Verification items for the finished model (mm, model axes). Face numbers are marked on the shaded views. A direction names the side the tool comes from. Coordinates: 2 decimals unless noted, no trailing zeros. Write each loop counter-clockwise with the first axis right and the second up, starting at its lowest first coordinate (ties: lowest second). Pieces come first, ordered by that corner, then holes. Notation, with made-up numbers: M 50,23 L 66,23 A13 cw 66,44 Z; hole C -27,6 d3. An arc over 180 degrees is marked long. Answer in a Markdown table with one row per item.
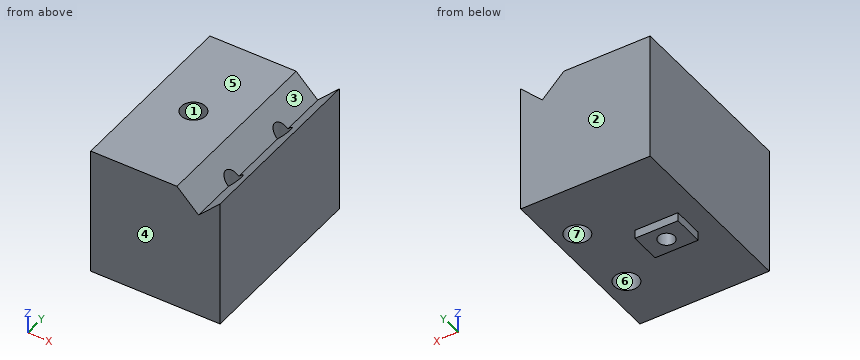
from build123d import *

# Parameters (mm, degrees)
F0_W      = 76.2
F0_H      = 76.2
F1_DEPTH  = 53.975
F3_DEPTH  = 107.951
F5_W      = 18.288
F5_H      = 5.08
F6_DEPTH  = 63.5
F4_R      = 4.7625
F7_DEPTH  = 81.281
F8_R      = 7.1501
F9_DEPTH  = 12.7
F10_R     = 7.1501
F11_DEPTH = 12.7
F12_W     = 38.1
F12_H     = 9
F13_DEPTH = 107.951


with BuildPart() as f1:
    # F0 (on Front) → F1 (new body, symmetric)
    with BuildSketch(Plane.XZ):
        with Locations((0, 38.1)):
            Rectangle(F0_W, F0_H)
    extrude(amount=F1_DEPTH, both=True)

    # F2 (on face) → F3 (cut, through all)
    with BuildSketch(Plane.XZ.offset(53.975)):
        Polygon((38.1, 76.2), (12.7, 76.2), (25.4, 63.5), align=None)
    extrude(amount=-F3_DEPTH, mode=Mode.SUBTRACT)

    # F5 (on face) → F6 (join)
    with BuildSketch(Plane.YZ.offset(38.1)):
        with Locations((0, -2.54)):
            Rectangle(F5_W, F5_H)
    extrude(amount=-F6_DEPTH)

    # F4 (on face) → F7 (cut, through all)
    with BuildSketch(Plane.XY.offset(76.2)):
        with Locations((25.4, 22.225)):
            Circle(F4_R)
        with Locations((25.4, -22.225)):
            Circle(F4_R)
        with Locations((-12.7, 0)):
            Circle(F4_R)
    extrude(amount=-F7_DEPTH, mode=Mode.SUBTRACT)

    # F8 (on face) → F9 (cut)
    with BuildSketch(Plane(origin=(0, 0, 0), x_dir=(1, 0, 0), z_dir=(0, 0, -1))):
        with Locations((25.4, -22.225)):
            Circle(F8_R)
        with Locations((25.4, 22.225)):
            Circle(F8_R)
    extrude(amount=-F9_DEPTH, mode=Mode.SUBTRACT)

    # F10 (on face) → F11 (cut)
    with BuildSketch(Plane.XY.offset(76.2)):
        with Locations((-12.7, 0)):
            Circle(F10_R)
    extrude(amount=-F11_DEPTH, mode=Mode.SUBTRACT)

    # F12 (on face) → F13 (cut, through all)
    with BuildSketch(Plane.XZ.offset(53.975)):
        with Locations((19.05, -4.5)):
            Rectangle(F12_W, F12_H)
    extrude(amount=-F13_DEPTH, mode=Mode.SUBTRACT)


solid = f1.part
1) Release check for a two-part mould opening along Y. For the marked faces 4, 5, 6 and 7 record: +Y half, -Y half, draft (parallel to the pull), parting line (faces both ways), or undercut.
Response values:
| item | result |
|---|---|
| face 4 | -Y half |
| face 5 | draft |
| face 6 | undercut |
| face 7 | undercut |
2) Sectioned sample at D-D (x = -21.5). Record the cut outline in (y, z) (3 decimals).
Response values:
| item | result |
|---|---|
| outline | M -53.975,0 L -9.144,0 L -9.144,-5.08 L 9.144,-5.08 L 9.144,0 L 53.975,0 L 53.975,76.2 L -53.975,76.2 Z |
3) Depth check by flat-ended pin: pin 1 (2.5 mm diameter, centred on y = -2, z = -2.5, fed in from -X); pin 2 (4.5 mm diameter, centred on x = 27.5, y = -19.5, fed in from -Z); pin 3 (15 mm diameter, centred on x = -12.7, y = 0, fed in from +Z); pin 4 (1.5 mm diameter, centred on x = 19.5, y = 16.5, fed in from -Z). Enter the tip coordinate at first touch or a pass-through.
Response values:
| item | result |
|---|---|
| pin 1 | stops at x = -25.4 |
| pin 2 | stops at z = 12.7 |
| pin 3 | stops at z = 76.2 |
| pin 4 | stops at z = 0 |
4) Sectioned sample at C-C (x = -12.7). Record the cut outline in (y, z) (1 decimal).
Response values:
| item | result |
|---|---|
| outline | M -54,0 L -9.1,0 L -9.1,-5.1 L -4.8,-5.1 L -4.8,63.5 L -7.2,63.5 L -7.2,76.2 L -54,76.2 Z; M 4.8,-5.1 L 9.1,-5.1 L 9.1,0 L 54,0 L 54,76.2 L 7.2,76.2 L 7.2,63.5 L 4.8,63.5 Z |
5) Sectioned sample at A-A (y = 0). Record the cut outline in (x, z).
Response values:
| item | result |
|---|---|
| outline | M -38.1,0 L -25.4,0 L -25.4,-5.08 L -17.46,-5.08 L -17.46,63.5 L -19.85,63.5 L -19.85,76.2 L -38.1,76.2 Z; M -7.94,-5.08 L 0,-5.08 L 0,0 L 38.1,0 L 38.1,76.2 L 25.4,63.5 L 12.7,76.2 L -5.55,76.2 L -5.55,63.5 L -7.94,63.5 Z |
6) Sectioned sample at B-B (z = 65). Record the cut outline in (x, y) (1 decimal), then the cut area to 4 significant figures.
Response values:
| item | result |
|---|---|
| outline | M -38.1,-54 L 23.9,-54 L 23.9,-26.7 A4.8 cw 23.9,-17.7 L 23.9,17.7 A4.8 cw 23.9,26.7 L 23.9,54 L -38.1,54 Z; M 26.9,-54 L 38.1,-54 L 38.1,54 L 26.9,54 L 26.9,26.7 A4.8 cw 26.9,17.7 L 26.9,-17.7 A4.8 cw 26.9,-26.7 Z; hole C -12.7,0 d14.3 |
| area | 7,655 mm² |
7) Tool access check on the marked faces 1, 2 and 3. Record the directions out of +Z, -Z, +X, -X, +Y, -Y that give a thin tool (end or side, any length) a straight path to the whole face; none if there is none.
Response values:
| item | result |
|---|---|
| face 1 | +Z |
| face 2 | +Z, -Z, +X, -X, +Y |
| face 3 | +Z, +Y, -Y |
8) Thickness scan on L1, parallel to Y at x = 25, z = 48 (3 decimals); L2, parallel to Y at x = 25, z = 8 (3 decimals); L3, parallel to Y at x = -12.7, z = 71.25 (3 decimals). Record the ranges inside material, lowest first. Write a range as [from, to].
Response values:
| item | result |
|---|---|
| L1 | y = [-53.975, -26.971], [-17.479, 17.479], [26.971, 53.975] |
| L2 | y = [-53.975, -29.364], [-15.086, 15.086], [29.364, 53.975] |
| L3 | y = [-53.975, -7.15], [7.15, 53.975] |
